CAD build for the part. Positions are in the model's coordinates, mm. A direction names the side the tool comes from. Give positions to 0.01 mm unless a question says otherwise; leave off trailing zeros. Write each loop counter-clockwise with the first axis right and the second up, starting at its lowest first coordinate (ties: lowest second). Pieces come first, ordered by that corner, then holes. Notation, with made-up numbers: (22.5, 84.25) -> (59.5, 84.25) arc R23 cw to (59.5, 106.25) -> close; hole circle Ø3 at (-16, 19.5). An arc over 180 degrees is marked (long way). Use one line per item in the form item = value. Start each with the question number.
from build123d import *

# Parameters (mm, degrees)
F0_W           = 33.2969208248
F0_H           = 32.5569906272
F1_DEPTH       = 30
F3_DEPTH       = 10
F5_D           = 12
F6_D           = 3
F6_CBORE_D     = 5
F6_CBORE_DEPTH = 2
F8_W           = 33.2969208248
F8_H           = 31.3508008987
F9_DEPTH       = 10


with BuildPart() as f1:
    # F0 (on Top) → F1 (new body)
    with BuildSketch(Plane.XY):
        with Locations((-11.1816951539, -9.1013486963)):
            Rectangle(F0_W, F0_H)
    extrude(amount=F1_DEPTH)

    # F2 (on face) → F3 (join)
    with BuildSketch(Plane.XY.offset(30)):
        Polygon((-15.3242121898, -16.2763986737), (-7.039178118, -16.2763986737), (-2.8966610822, -9.1013486963), (-7.039178118, -1.9262987189), (-15.3242121898, -1.9262987189), (-19.4667292257, -9.1013486963), align=None)
        Polygon((-14.4506519977, -14.8810296934), (-17.8215241451, -9.1601895243), (-14.5525673013, -3.3805085272), (-7.9127383102, -3.3216676992), (-4.5418661628, -9.0425078683), (-7.8108230065, -14.8221888654), align=None, mode=Mode.SUBTRACT)
    extrude(amount=F3_DEPTH)

    # F5 (through all)
    with Locations(Plane.YZ.offset(5.4667652585)):
        with Locations((-10.5295337308, 16.1808457948)):
            Hole(F5_D / 2)

    # F6 (through all)
    with Locations(Plane.YZ.offset(5.4667652585)):
        with Locations((-20.3798440099, 25)):
            CounterBoreHole(F6_D / 2, F6_CBORE_D / 2, F6_CBORE_DEPTH)

    # F8 (on 3pt) → F9 (join)
    with BuildSketch(Plane(origin=(0, 6.5719923281, 1.994259097), x_dir=(1, 0, 0), z_dir=(0, -0.9569133528, -0.2903736133))):
        with Locations((-11.1816951539, 13.591346453)):
            Rectangle(F8_W, F8_H)
    extrude(amount=-F9_DEPTH)


solid = f1.part
1) Cut at B-B (x = -0.5). Give the cut face in (y, z).
2) Cut at A-A (z = 36). Give the cut face in (x, y), and give its area (3 significant figures).
3) Cut at C-C (y = -14). Give the cut face in (x, z), and give its area (3 significant figures).
4) Two-plate mould, pull along Y, no slides. Class faces 1 (the face through (-11.41, -6.11, 20.24)), 2 (the face through (5.467, -4, 16)), 3 (the face through (-11, -16.276, 35)), 4 (the face through (-11.41, 12.13, 18.11)): released by +Y, released by -Y, zero draft, split by the parting line, or undercut.
5) Cut at D-D (z = 25). Give the cut face in (x, y).
6) 3-axis set-ups, long thin cutter, end or side, ignore diameter. For faces 5 (the face through (-16.21, -6.31, 34.93)), 6 (the face through (4.48, -19.04, 27.11)), 7 (the face through (-17.366, -5.464, 34.93)), 8 (the face through (-11, -1.926, 35)): which of +Z, -Z, +X, -X, +Y, -Y reach the whole face in a straight line?
7) Wall check: line 1 along X through (y, z) = (-19, 23); line 2 along Y through (x, z) = (-25, 25.5); line 3 along Z through (x, y) = (-19.5, -18). Give the ranges that are in metal, low to high. Write a range as from..to.
8) Pin check, flat tips, straight feed: pin 1 (4 mm diameter, centred on y = -20, z = 25.5, fed in from +X); pin 2 (8 mm diameter, centred on x = -6, y = 3.5, fed in from +Z); pin 3 (4 mm diameter, centred on y = -20.38, z = 25, fed in from +X); pin 4 (5 mm diameter, centred on x = -10, y = 11, fed in from -Z). Stop position of each tip, or through.
Final values:
q1.outline = (-25.38, 0) -> (7.18, 0) -> (16.75, 2.9) -> (7.64, 32.9) -> (-1.93, 30) -> (-25.38, 30) -> close; hole circle Ø3 at (-20.38, 25); hole circle Ø12 at (-10.53, 16.18)
q2.outline = (-19.47, -9.1) -> (-15.32, -16.28) -> (-7.04, -16.28) -> (-2.9, -9.1) -> (-7.04, -1.93) -> (-15.32, -1.93) -> close; hole (-17.82, -9.16) -> (-14.45, -14.88) -> (-7.81, -14.82) -> (-4.54, -9.04) -> (-7.91, -3.32) -> (-14.55, -3.38) -> close
q2.area = 63.8 mm^2
q3.outline = (-27.83, 0) -> (5.47, 0) -> (5.47, 11.29) -> (-27.83, 11.29) -> close; (-27.83, 21.08) -> (5.47, 21.08) -> (5.47, 30) -> (-5.72, 30) -> (-5.72, 40) -> (-7.35, 40) -> (-7.35, 30) -> (-14.97, 30) -> (-14.97, 40) -> (-16.64, 40) -> (-16.64, 30) -> (-27.83, 30) -> close
q3.area = 706 mm^2
q4.face_1 = undercut
q4.face_2 = zero draft
q4.face_3 = released by -Y
q4.face_4 = released by +Y
q5.outline = (-27.83, -25.38) -> (5.47, -25.38) -> (5.47, -22.88) -> (3.47, -22.88) -> (3.47, -21.88) -> (-27.83, -21.88) -> close; (-27.83, -18.88) -> (3.47, -18.88) -> (3.47, -17.88) -> (5.47, -17.88) -> (5.47, 10.04) -> (-27.83, 10.04) -> close
q6.face_5 = +Z
q6.face_6 = +X
q6.face_7 = +Z, -X
q6.face_8 = +Z, +X, -X
q7.line_1 = -27.83..3.47
q7.line_2 = -25.38..-21.79, -18.97..9.89
q7.line_3 = 0..30
q8.pin_1 = 5.47
q8.pin_2 = 32.86
q8.pin_3 = 3.47
q8.pin_4 = 0.4
